from build123d import *

# Parameters (mm, degrees)
F0_W     = 30.0332503393
F0_H     = 3.0297264457
F1_DEPTH = 15
F0_W_2   = 36.8763273582
F0_H_2   = 1.4379325638
F2_DEPTH = 7.5
F3_SIZE2 = 7.49999
F3_SIZE  = 9.99999
F4_SIZE2 = 7.49999
F4_SIZE  = 9.99999


# Not quite as in the source:
# - a fillet or chamfer is up to 0.001 mm smaller than in the source, because OpenCascade refuses the exact size


with BuildPart() as f1:
    # F0 (on Top) → F1 (new body, symmetric)
    with BuildSketch(Plane.XY):
        with Locations((-4.9947178923, 25.5465358496)):
            Rectangle(F0_W, F0_H)
    extrude(amount=F1_DEPTH, both=True)

    # F0 (on Top) → F2 (join, symmetric)
    with BuildSketch(Plane.XY):
        with Locations((-4.9947178923, 25.5465358496)):
            Rectangle(F0_W, F0_H)
        with Locations((28.4600709565, 27.7803653543)):
            Rectangle(F0_W_2, F0_H_2)
        with Locations((28.4600709565, 25.5465358496)):
            Rectangle(F0_W_2, F0_H)
        with BuildLine():
            ThreePointArc((46.8982346356, -58.3157722523), (89.586820298, -15.62718659), (46.8982346356, 27.0613990724))
            Line((46.8982346356, 27.0613990724), (46.8982346356, 24.0316726267))
            ThreePointArc((46.8982346356, 24.0316726267), (86.5570938523, -15.62718659), (46.8982346356, -55.2860458066))
            Line((46.8982346356, -55.2860458066), (46.8982346356, -58.3157722523))
        make_face()
        with BuildLine():
            Line((46.8982346356, 28.4993316362), (46.8982346356, 27.0613990724))
            ThreePointArc((46.8982346356, 27.0613990724), (89.586820298, -15.62718659), (46.8982346356, -58.3157722523))
            Line((46.8982346356, -58.3157722523), (46.8982346356, -59.7537048161))
            ThreePointArc((46.8982346356, -59.7537048161), (91.0247528617, -15.62718659), (46.8982346356, 28.4993316362))
        make_face()
    extrude(amount=F2_DEPTH, both=True)

    # F3 (size 10 and 7.5 in the source; OpenCascade refuses exactly that, so slightly less here)
    f3_edges = [f1.edges().sort_by_distance(p)[0] for p in [
        (10.021907, 25.546536, 7.5),
    ]]
    f3_side = f1.faces().sort_by_distance((11.219825, 27.780365, 7.5))[0]
    chamfer(f3_edges, length=F3_SIZE, length2=F3_SIZE2, reference=f3_side)

    # F4 (size 10 and 7.5 in the source; OpenCascade refuses exactly that, so slightly less here)
    f4_edges = [f1.edges().sort_by_distance(p)[0] for p in [
        (10.021907, 25.546536, -7.5),
    ]]
    f4_side = f1.faces().sort_by_distance((11.219825, 27.780365, -7.5))[0]
    chamfer(f4_edges, length=F4_SIZE, length2=F4_SIZE2, reference=f4_side)


solid = f1.part
Input: part model. Units: mm. Frame: model coordinates. A direction names the side the tool comes from. Coordinates: 2 decimals unless noted, no trailing zeros. Order: outer loops, then holes, each group sorted by start corner. A loop starts at its lowest first (then second) coordinate and runs counter-clockwise, first axis right, second up.
1. Cut plane A-A, the plane x = 52.5. Return loops of the section in (y, z), plus the area to 3 significant figures.
Checked values:
outline: (-59.4, -7.5) - (-54.89, -7.5) - (-54.89, 7.5) - (-59.4, 7.5) - close; (23.63, -7.5) - (28.14, -7.5) - (28.14, 7.5) - (23.63, 7.5) - close
area: 135 mm2
2. Access query for faces 5 (the flat face through (14.952, 25.568, 11.302)), 6 (the flat face through (46.898, -57, 0)). Directions: +Z, -Z, +X, -X, +Y, -Y. A direction counts if a zero-diameter tool reaches every point of the face in a straight line with its end or side. Return the directions, or none.
Checked values:
face 5: +Z, +X, +Y, -Y
face 6: +Z, -Z, -X, -Y
3. Cut plane C-C, the plane x = 24. Return loops of the section in (y, z).
Checked values:
outline: (24.03, -7.5) - (28.5, -7.5) - (28.5, 7.5) - (24.03, 7.5) - close
4. Cut plane D-D, the plane y = 15. Return loops of the section in (x, z).
Checked values:
outline: (72.09, -7.5) - (78.66, -7.5) - (78.66, 7.5) - (72.09, 7.5) - close
5. Contact query for flat-ended pins moving along their axis: P1, Ø8, axis at y = -25.5, z = -3.5, coming from the +X side; P2, Ø1, axis at y = -43.5, z = -1, coming from the -X side; P3, Ø15, axis at x = -6.5, z = -1, coming from the +Y side. Output: stop coordinate, or through.
Checked values:
P1: stops at x = 90.63
P2: stops at x = 74.61
P3: stops at y = 27.06
6. Draft query along Y for faces 1 (the flat face through (-5, 27.061, 0)), 2 (the cylindrical face through (86.548, -14.755, 0.105)), 3 (the cylindrical face through (91.014, -16.598, 0.105)), 4 (the flat face through (83.3, 0.9, -7.5)). Return one class per face: +Y half, -Y half, draft (parallel to the pull), parting line (faces both ways), or undercut.
Checked values:
face 1: +Y half
face 2: undercut
face 3: parting line
face 4: draft
7. Ray query, line 1 along Y through (x, z) = (39, 5.5); line 2 along Y through (x, z) = (-3.5, -4.5); line 3 along Y through (x, z) = (51, 5.75). Return the intervals inside material, ascending.
Checked values:
line 1: y = 24.03 to 28.5
line 2: y = 24.03 to 27.06
line 3: y = -59.56 to -55.07, 23.82 to 28.31
